Can you work these out from the model? Positions are in its coordinate system, mm. A direction names the side the tool comes from. Give positions to 0.01 mm unless a question says otherwise; leave off trailing zeros. Write each loop counter-clockwise with the first axis right and the second up, starting at its lowest first coordinate (ties: lowest second). Pieces come first, ordered by that corner, then holes. Notation, with made-up numbers: (57, 14) -> (90, 14) arc R11 cw to (90, 25) -> close; hole circle Ø10 at (8, 65.5). An arc over 180 degrees is marked (long way). One line per item, written item: value.
Autodesk Inventor part; units mm, degrees
ref_plane "YZ Plane" through (0, 0, 0) normal (1, 0, 0) x (0, 1, 0)
ref_plane "XZ Plane" through (0, 0, 0) normal (0, 1, 0) x (-1, 0, 0)
ref_plane "XY Plane" through (0, 0, 0) normal (0, 0, 1) x (1, 0, 0)
sketch "Boceto1" plane through (0, 0, 0) normal (0, 0, 1) x (1, 0, 0)
  line L0 (0, 0) -> (164, 0)
  line L1 (164, 0) -> (164, 86)
  line L2 (164, 86) -> (0, 86)
  line L3 (0, 86) -> (0, 0)
  dimension "d0" = 164
  dimension "d1" = 86
extrude "Base" add sketch "Boceto1" along normal blind 82
sketch "Boceto2" plane through (0, 0, 82) normal (0, 0, 1) x (1, 0, 0)
  line L0 (0, 0) -> (164, 0)
  line L1 (164, 0) -> (134, 0)
  line L2 (134, 0) -> (134, 12)
  line L3 (134, 12) -> (164, 12)
  line L4 (164, 12) -> (164, 0)
  dimension "d4" = 30
  dimension "d5" = 12
extrude "Orificio_Inferior_Derecho" cut sketch "Boceto2" against normal blind 82
sketch "Boceto3" plane through (0, 0, 82) normal (0, 0, 1) x (1, 0, 0)
  line L0 (0, 86) -> (0, 0)
  line L1 (0, 0) -> (30, 0)
  line L2 (30, 0) -> (30, 12)
  line L3 (30, 12) -> (0, 12)
  line L4 (0, 12) -> (0, 0)
  dimension "d8" = 30
  dimension "d9" = 12
extrude "Orificio_Inferior_Izquierdo" cut sketch "Boceto3" against normal blind 82
sketch "Boceto5" plane through (0, 0, 0) normal (0, 0, -1) x (-1, 0, 0)
  line L0 (-164, 86) -> (0, 86)
  arc A0 (-116, 86) -> (-48, 86) centre (-82, 86) ccw
  point P0 (0, 0)
  dimension "d15" = 68
extrude "Medio_Círculo" cut sketch "Boceto5" against normal blind 34
sketch "Boceto7" plane through (0, 0, 82) normal (0, 0, 1) x (1, 0, 0)
  line L0 (0, 118.5619) -> (0, 23.764) construction
  line L1 (164, 118.5619) -> (164, 23.764) construction
  line L2 (164, 12) -> (164, 86)
  line L3 (0, 86) -> (0, 12)
  line L4 (202.848, 28) -> (-57.2499, 28) construction
  line L5 (30, 0) -> (134, 0)
  line L6 (164, 86) -> (0, 86)
  line L7 (0, 86) -> (164, 86)
  line L8 (164, 86) -> (164, 28)
  line L9 (164, 28) -> (0, 28)
  line L10 (0, 28) -> (0, 86)
  point P0 (0, 0)
  dimension "d23" = 0
  dimension "d24" = 0
  dimension "d25" = 28
extrude "Hueco" cut sketch "Boceto7" against normal blind 48
sketch "Boceto8" plane through (134, 0, 0) normal (0, -1, 0) x (1, 0, 0)
  line L0 (-150.3038, 58) -> (47.6348, 58) construction
  line L1 (-52, -16.1765) -> (-52, 95.9123) construction
  line L2 (30, 82) -> (30, 0)
  line L3 (-104, 82) -> (0, 82)
  circle A0 centre (-52, 58) radius 12
  point P0 (-134, 0)
  dimension "d28" = 82
  dimension "d29" = 24
  dimension "d30" = 24
extrude "Círculo" cut sketch "Boceto8" against normal blind 28
sketch "Boceto9" plane through (164, 12, 0) normal (1, 0, 0) x (0, 0, -1)
  line L0 (-92.1417, 50) -> (23.5619, 50) construction
  line L1 (-34, 16) -> (-82, 16)
  line L2 (-34, 74) -> (-34, 16)
  line L3 (-34, 50) -> (-82, 16)
  line L4 (-34, 16) -> (-34, 50)
  line L5 (-34, 16) -> (-82, 16)
  point P0 (0, -12)
  dimension "d33" = 34
extrude "Triángulo_Derecho" add sketch "Boceto9" against normal blind 20
sketch "Boceto10" plane through (0, 12, 0) normal (-1, 0, 0) x (0, 0, 1)
  line L0 (-15.7199, 50) -> (95.5491, 50) construction
  line L1 (82, 16) -> (34, 16)
  line L2 (34, 16) -> (34, 50)
  line L3 (34, 50) -> (34, 16)
  line L4 (82, 16) -> (34, 16)
  line L5 (34, 16) -> (82, 16)
  line L6 (82, 16) -> (34, 50)
  point P0 (0, -12)
  dimension "d36" = 34
extrude "Triángulo_Izquierdo" add sketch "Boceto10" against normal blind 20
sketch "Boceto11" plane through (0, 0, 0) normal (0, 0, -1) x (-1, 0, 0)
  line L0 (-144, 115.7571) -> (-144, -22.8513) construction
  line L1 (-164, 12) -> (-164, 86)
  line L2 (-189.9872, 62) -> (67.4285, 62) construction
  line L3 (-30, 0) -> (-134, 0)
  line L4 (-116, 86) -> (-164, 86)
  line L5 (-189.9872, 86) -> (-164, 86) construction
  line L6 (-197.4576, 74) -> (12.6853, 74) construction
  line L7 (-144, 86) -> (-164, 86)
  line L8 (-164, 86) -> (-164, 62)
  line L9 (-164, 86) -> (-164, 74)
  line L10 (-164, 74) -> (-144, 86)
  point P0 (0, 0)
  dimension "d39" = 20
  dimension "d40" = 62
  dimension "d41" = 24
  dimension "d42" = 12
extrude "Recorte_Superior_Derecho" cut sketch "Boceto11" against normal blind 34
sketch "Boceto12" plane through (0, 0, 0) normal (0, 0, -1) x (-1, 0, 0)
  line L0 (-163.8025, 74) -> (21.144, 74) construction
  line L1 (-20, 114.5089) -> (-20, -16.4312) construction
  line L2 (-48, 86) -> (0, 86)
  line L3 (0, 86) -> (0, 12)
  line L4 (0, 86) -> (-20, 86)
  line L5 (0, 62) -> (0, 86)
  line L6 (0, 74) -> (0, 86)
  line L7 (0, 86) -> (0, 74)
  line L8 (0, 74) -> (-20, 86)
  point P0 (0, 0)
  dimension "d45" = 12
  dimension "d46" = 20
extrude "Recorte_Superior_Izquierdo" cut sketch "Boceto12" against normal blind 34
1) We'd pull the mould along X, two halves only. Please class faces 1 (the face through (130, 86, 17)), 2 (the face through (134, 6, 42)), 3 (the face through (82.75, 52.01, 16.76)): released by +X, released by -X, zero draft, split by the parting line, or undercut.
Answer list:
face 1: zero draft
face 2: released by +X
face 3: undercut
2) For faces 4 (the face through (97, 28, 58)), 5 (the face through (81, 17, 82)), 6 (the face through (149, 12, 42)), 7 (the face through (15, 12, 42)), which set-ups out of +Z, -Z, +X, -X, +Y, -Y let a thin tool reach every point of the face, with its end or its side?
Answer list:
face 4: +Z, +Y
face 5: +Z, +X, -X, +Y, -Y
face 6: +Z, -Z, +X, -Y
face 7: +Z, -Z, -X, -Y
3) I need wall thicknesses on L1, parallel to Z at x = 82, y = 22; L2, parallel to X at y = 47, z = 42; L3, parallel to Z at x = 119, y = 68. Which ranges of each line are inside material? Lowest first, please.
Answer list:
L1: z = 0 to 46, 70 to 82
L2: x = 0 to 20, 144 to 164
L3: z = 0 to 34
4) If we section it at B-B (z = 67.5): Write out the boundary of the cut face in (x, y), and give its area (3 significant figures).
Answer list:
outline: (0, 12) -> (30, 12) -> (30, 0) -> (74.67, 0) -> (74.67, 28) -> (20, 28) -> (20, 38.27) -> (0, 38.27) -> close; (89.33, 0) -> (134, 0) -> (134, 12) -> (164, 12) -> (164, 38.27) -> (144, 38.27) -> (144, 28) -> (89.33, 28) -> close
area: 3,870 mm^2
5) Will these pins go through, and if not, where does the flat tip stop? pin 1 (14.5 mm diameter, centred on x = 82, z = 58, fed in from +Y); pin 2 (9.5 mm diameter, centred on y = 3.5, z = 34.5, fed in from +X); pin 3 (12 mm diameter, centred on x = 146, y = 74.5, fed in from +Z); pin 4 (4 mm diameter, centred on x = 70.5, z = 52.5, fed in from +Y).
Answer list:
pin 1: passes through
pin 2: stops at x = 134
pin 3: stops at z = 34
pin 4: stops at y = 28
6) If we section it at D-D (y = 71): Write out the boundary of the cut face in (x, z), and give its area (3 significant figures).
Answer list:
outline: (0, 0) -> (51.49, 0) -> (51.49, 34) -> (0, 34) -> close; (112.51, 0) -> (164, 0) -> (164, 34) -> (112.51, 34) -> close
area: 3,500 mm^2
7) If we section it at C-C (y = 26): Write out the boundary of the cut face in (x, z), and give its area (3 significant figures).
Answer list:
outline: (0, 0) -> (164, 0) -> (164, 82) -> (0, 82) -> close; hole circle Ø24 at (82, 58)
area: 13,000 mm^2
8) If we section it at A-A (x = 82): Write out the boundary of the cut face in (y, z).
Answer list:
outline: (0, 0) -> (52, 0) -> (52, 34) -> (28, 34) -> (28, 46) -> (0, 46) -> close; (0, 70) -> (28, 70) -> (28, 82) -> (0, 82) -> close
